Here's how the part is built. I have some questions about the finished solid (model axes, mm). Face numbers are marked on the shaded views. Round coordinates to 2 decimals unless told otherwise and drop trailing zeros. Loops run counter-clockwise (first coordinate to the right, second up) from the corner with the lowest first, then second, coordinate; pieces in that order, holes last. Notation, with made-up numbers: M 36.5,34.5 L 54.5,34.5 A25 cw 54.5,49.5 Z; hole C 76.5,-19.75 d8. An arc over 180 degrees is marked long. Answer as a JSON object with one key per item and string values.
from build123d import *

# Parameters (mm, degrees)
F0_W     = 4.5
F0_H     = 27.8
F0_R     = 1.6
F1_DEPTH = 7
F2_SIZE  = 5


with BuildPart() as f1:
    # F0 (on Top) → F1 (new body)
    with BuildSketch(Plane.XY):
        Rectangle(F0_W, F0_H)
        Circle(F0_R, mode=Mode.SUBTRACT)
    extrude(amount=F1_DEPTH)

    # F2
    f2_edges = [f1.edges().sort_by_distance(p)[0] for p in [
        (0, -13.9, 7),
        (0, 13.9, 7),
    ]]
    chamfer(f2_edges, length=F2_SIZE)


solid = f1.part
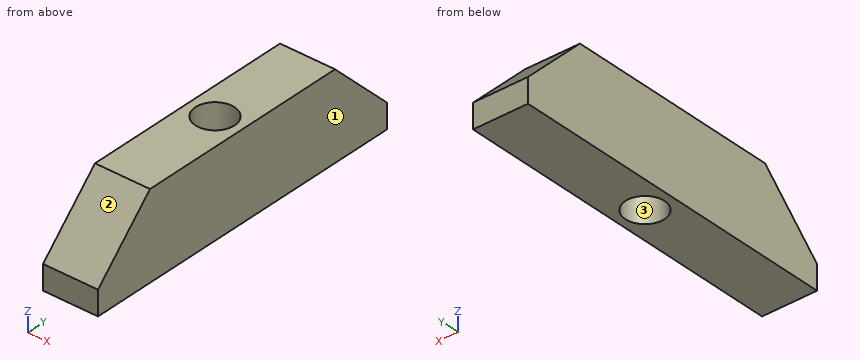
Item 1: If I drill on L1, parallel to Y at x = 0, z = 1.5; L2, parallel to Y at x = 0, z = 2.75; L3, parallel to X at y = 1.25, z = 3.25, over which ranges is the centre line in solid material (lowest first)? Write a range as from..to.
Solution:
{"L1": "y = -13.9..-1.6, 1.6..13.9", "L2": "y = -13.15..-1.6, 1.6..13.15", "L3": "x = -2.25..-1, 1..2.25"}
Item 2: I want a section at B-B on z = 6. List the corners of the cut face in (x, y) for me, plus the area to 3 significant figures.
Solution:
{"outline": "M -2.25,-9.9 L 2.25,-9.9 L 2.25,9.9 L -2.25,9.9 Z; hole C 0,0 d3.2", "area": "81.1 mm2"}
Item 3: I want a section at C-C on x = 0. List the corners of the cut face in (y, z) for me.
Solution:
{"outline": "M -13.9,0 L -1.6,0 L -1.6,7 L -8.9,7 L -13.9,2 Z; M 1.6,0 L 13.9,0 L 13.9,2 L 8.9,7 L 1.6,7 Z"}
Item 4: I want a section at A-A on y = 0. List the corners of the cut face in (x, z) for me.
Solution:
{"outline": "M -2.25,0 L -1.6,0 L -1.6,7 L -2.25,7 Z; M 1.6,0 L 2.25,0 L 2.25,7 L 1.6,7 Z"}
Item 5: I want a section at D-D on z = 4.5. List the corners of the cut face in (x, y) for me.
Solution:
{"outline": "M -2.25,-11.4 L 2.25,-11.4 L 2.25,11.4 L -2.25,11.4 Z; hole C 0,0 d3.2"}
Item 6: We'd pull the mould along X, two halves only. Please class the marked faces 1, 2 and 3: +X half, -X half, draft (parallel to the pull), parting line (faces both ways), or undercut.
Solution:
{"face 1": "+X half", "face 2": "draft", "face 3": "undercut"}
Item 7: For P1, Ø1, axis at x = -0.5, y = 4.5, coming from the -Z side; P2, Ø1.5, axis at x = -1.5, z = 4.5, coming from the -Y side, each with a flat end and sliding along its axis, tell me the tip position at first contact or that it passes through.
Solution:
{"P1": "stops at z = 0", "P2": "stops at y = -12.15"}
